Verification items for the finished model (mm, model axes). Coordinates: 2 decimals unless noted, no trailing zeros. Write each loop counter-clockwise with the first axis right and the second up, starting at its lowest first coordinate (ties: lowest second). Pieces come first, ordered by that corner, then holes. Notation, with made-up numbers: (63, 50) -> (120, 50) arc R14 cw to (120, 72) -> close; hole circle Ø2 at (15, -38.5). An arc over 180 degrees is marked (long way). Answer in a Markdown table with one row per item.
```python
from build123d import *

# Parameters (mm, degrees)
SKETCH1_R           = 4.445
SKETCH1_R_2         = 3.175
SKETCH1_R_3         = 2.794
SKETCH1_W           = 25.4
SKETCH1_H           = 6.35
BOSS_EXTRUDE1_DEPTH = 6.35


with BuildPart() as part:
    # Sketch1 → Boss-Extrude1 (new body)
    with BuildSketch(Plane(origin=(0, 0, 0), x_dir=(1, 0, 0), z_dir=(0, 1, 0))):
        with BuildLine():
            Line((50.8, 0), (463.677487426, 0))
            ThreePointArc((463.677487426, 0), (499.59851191, 14.878975516), (514.477487426, 50.8))
            Line((514.477487426, 50.8), (514.477487426, 279.4))
            ThreePointArc((514.477487426, 279.4), (507.037999668, 297.360512242), (489.077487426, 304.8))
            Line((489.077487426, 304.8), (25.4, 304.8))
            ThreePointArc((25.4, 304.8), (7.439487758, 297.360512242), (0, 279.4))
            Line((0, 279.4), (0, 50.8))
            ThreePointArc((0, 50.8), (14.878975516, 14.878975516), (50.8, 0))
        make_face()
        with Locations((305.32695, 213.055054)):
            Circle(SKETCH1_R, mode=Mode.SUBTRACT)
        with Locations((305.32695, 71.425054)):
            Circle(SKETCH1_R, mode=Mode.SUBTRACT)
        with Locations((502.173875, 116.4574125)):
            Circle(SKETCH1_R_2, mode=Mode.SUBTRACT)
        with Locations((502.173875, 188.2917875)):
            Circle(SKETCH1_R_2, mode=Mode.SUBTRACT)
        with Locations((12.303125, 116.4574125)):
            Circle(SKETCH1_R_2, mode=Mode.SUBTRACT)
        with Locations((12.303125, 188.2917875)):
            Circle(SKETCH1_R_2, mode=Mode.SUBTRACT)
        with Locations((209.27695, 71.425054)):
            Circle(SKETCH1_R, mode=Mode.SUBTRACT)
        with Locations((209.27695, 213.055054)):
            Circle(SKETCH1_R, mode=Mode.SUBTRACT)
        with Locations((221.3848125, 50.403125)):
            Circle(SKETCH1_R_2, mode=Mode.SUBTRACT)
        with Locations((221.3848125, 12.303125)):
            Circle(SKETCH1_R_2, mode=Mode.SUBTRACT)
        with Locations((293.2191875, 50.403125)):
            Circle(SKETCH1_R_2, mode=Mode.SUBTRACT)
        with Locations((293.2191875, 12.303125)):
            Circle(SKETCH1_R_2, mode=Mode.SUBTRACT)
        with Locations((147.3962, 177.7746)):
            Circle(SKETCH1_R_2, mode=Mode.SUBTRACT)
        with Locations((147.3962, 126.9746)):
            Circle(SKETCH1_R_2, mode=Mode.SUBTRACT)
        with Locations((147.3962, 152.3746)):
            Circle(SKETCH1_R_2, mode=Mode.SUBTRACT)
        with Locations((367.081287426, 152.3746)):
            Circle(SKETCH1_R_2, mode=Mode.SUBTRACT)
        with Locations((367.081287426, 126.9746)):
            Circle(SKETCH1_R_2, mode=Mode.SUBTRACT)
        with Locations((367.081287426, 177.7746)):
            Circle(SKETCH1_R_2, mode=Mode.SUBTRACT)
        with Locations((497.175487426, 244.4496)):
            Circle(SKETCH1_R_3, mode=Mode.SUBTRACT)
        with Locations((377.175487426, 244.4496)):
            Circle(SKETCH1_R_3, mode=Mode.SUBTRACT)
        with Locations((137.175487426, 244.4496)):
            Circle(SKETCH1_R_3, mode=Mode.SUBTRACT)
        with Locations((17.175487426, 244.4496)):
            Circle(SKETCH1_R_3, mode=Mode.SUBTRACT)
        with Locations((498.475487426, 231.7496)):
            Rectangle(SKETCH1_W, SKETCH1_H, mode=Mode.SUBTRACT)
        with Locations((422.275487426, 231.7496)):
            Rectangle(SKETCH1_W, SKETCH1_H, mode=Mode.SUBTRACT)
        with Locations((346.075487426, 231.7496)):
            Rectangle(SKETCH1_W, SKETCH1_H, mode=Mode.SUBTRACT)
        with Locations((168.275487426, 231.7496)):
            Rectangle(SKETCH1_W, SKETCH1_H, mode=Mode.SUBTRACT)
        with Locations((92.075487426, 231.7496)):
            Rectangle(SKETCH1_W, SKETCH1_H, mode=Mode.SUBTRACT)
        with Locations((15.875487426, 231.7496)):
            Rectangle(SKETCH1_W, SKETCH1_H, mode=Mode.SUBTRACT)
    extrude(amount=BOSS_EXTRUDE1_DEPTH)


solid = part.part
```
1. Depth check by flat-ended pin: P1, Ø4, axis at x = 367.08, z = -177.77, coming from the +Y side; P2, Ø3, axis at x = 22, y = 4.5, coming from the -Z side. Enter the tip coordinate at first touch or a pass-through.
Geometry says:
| item | result |
|---|---|
| P1 | through |
| P2 | z = -304.73 |
2. Thickness scan on line 1 (Z direction, x = 304.5, y = 5.75); line 2 (X direction, y = 3, z = -244.5); line 3 (X direction, y = 3, z = -127). Record the ranges inside material, lowest first. Write a range as from..to.
Geometry says:
| item | result |
|---|---|
| line 1 | -304.8..-217.42, -208.69..-75.79, -67.06..0 |
| line 2 | 0..14.38, 19.97..134.38, 139.97..374.38, 379.97..494.38, 499.97..514.48 |
| line 3 | 0..144.22, 150.57..363.91, 370.26..514.48 |
3. Section check A-A, the plane x = 85.5. Record the boundary of the cut face in (y, z), plus the area to 3 significant figures.
Geometry says:
| item | result |
|---|---|
| outline | (0, -304.8) -> (6.35, -304.8) -> (6.35, -234.92) -> (0, -234.92) -> close; (0, -228.57) -> (6.35, -228.57) -> (6.35, 0) -> (0, 0) -> close |
| area | 1,900 mm^2 |
4. Section check B-B, the plane y = 1.5. State how many separate pieces and enclosed holes the cut face has, plus the area to 3 significant figures.
Geometry says:
| item | result |
|---|---|
| separate pieces | 1 |
| enclosed holes | 28 |
| area | 154,000 mm^2 |
